Here's how the part is built. I have some questions about the finished solid (model axes, mm). A direction names the side the tool comes from. Coordinates: 2 decimals unless noted, no trailing zeros. Loops run counter-clockwise (first coordinate to the right, second up) from the corner with the lowest first, then second, coordinate; pieces in that order, holes last. Notation, with made-up numbers: (84.5, -1.75) -> (109.5, -1.75) arc R18 ccw to (109.5, 11.25) -> close; hole circle Ø11 at (30, -11). An arc over 180 degrees is marked (long way). Answer as a JSON object with one key per item and string values. Group by question number.
1) I want a section at C-C (z = 4). Count the separate pieces of the cut face and the enclosed holes in it, then the cut area to 3 significant figures.
2) If we mould it in two halves opening along X, with no side actions, what happens to faces 1 (the cylindrical face through (179.66, -8.5, 4.7)), 2 (the flat face through (80, 45, 0)), 3 (the flat face through (75.101, 119, 5))? For each: +X half, -X half, draft (parallel to the pull), parting line (faces both ways), or undercut.
3) I want a section at A-A (x = 172.5). Write out the boundary of the cut face in (y, z) (3 decimals), then the cut area to 3 significant figures.
4) I'm going to push flat-ended pins straight in: pin 1 (4 mm diameter, centred on y = 92.5, z = 5, fed in from -X); pin 2 (7.5 mm diameter, centred on x = -57.29, y = -9.46, fed in from -Z); pin 3 (0.9 mm diameter, centred on y = -45, z = 6.5, fed in from +X); pin 4 (3 mm diameter, centred on x = 120.5, z = 4, fed in from -Y). Where does each tip first touch, or does it pass through?
5) I need wall thicknesses on probe 1 along X at (y, z) = (-7, 6); probe 2 along Y at (x, z) = (83, 1.25); probe 3 along X at (y, z) = (-10, 6). Which ranges of each line are inside material? Lowest first, please. Write a range as [from, to].
6) I want a section at D-D (y = 120). Write out the boundary of the cut face in (x, z) (3 decimals), then the cut area to 3 significant figures.
7) Which directions (+Z, -Z, +X, -X, +Y, -Y) give clear straight access to the entire face, cutting with the end or side of a thin tool? Please do faces 4 (the flat face through (88, -44.322, 5)), 5 (the flat face through (-33, 80.741, 5)), 6 (the flat face through (222.711, 43, 5)).
8) I want a section at B-B (y = 66). Write out the boundary of the cut face in (x, z) (3 decimals).
```python
from build123d import *

# Parameters (mm, degrees)
SKETCH1_R                    = 14.2875
BOSS_EXTRUDE1_DEPTH          = 9.525
SKETCH2_W                    = 285.640227578
SKETCH2_H                    = 77.156349518
CUT_EXTRUDE1_DEPTH           = 267.58430025
SKETCH4_W                    = 213.36
SKETCH4_H                    = 65.465352004
CUT_EXTRUDE2_DEPTH           = 267.58430025
FILLET2_R                    = 25.4
SKETCH16_W                   = 9.525
SKETCH16_H                   = 0.985363282
CUT_EXTRUDE3_DEPTH           = 390.572219806
SKETCH17_W                   = 147.610011278
SKETCH17_H                   = 12.7
CUT_EXTRUDE4_DEPTH           = 267.045158533
TAP_DRILL_FOR_M6X0_75_TAP1_D = 5.25
F_6_4_6_4_DIAMETER_HOLE1_D   = 6.4


with BuildPart() as part:
    # Sketch1 → Boss-Extrude1 (new body)
    with BuildSketch(Plane.XY):
        Polygon((-138.259383474, 48.991487021), (32.210627804, -121.478524257), (222.710627804, -121.478524257), (222.710627804, 146.206839025), (-138.259383474, 146.206839025), align=None)
        with Locations(Location((180.538014078, 76.831975743, 0), (0, 0, 180))):
            Circle(SKETCH1_R, mode=Mode.SUBTRACT)
    extrude(amount=BOSS_EXTRUDE1_DEPTH)

    # Sketch2 → Cut-Extrude1 (cut, through all)
    with BuildSketch(Plane.XY.offset(9.525)):
        with Locations((98.940514015, -82.900349498)):
            Rectangle(SKETCH2_W, SKETCH2_H)
    extrude(amount=-CUT_EXTRUDE1_DEPTH, mode=Mode.SUBTRACT)

    # Sketch4 → Cut-Extrude2 (cut, through all)
    with BuildSketch(Plane.XY.offset(9.525)):
        with Locations((-31.579383474, 113.474163023)):
            Rectangle(SKETCH4_W, SKETCH4_H)
    extrude(amount=-CUT_EXTRUDE2_DEPTH, mode=Mode.SUBTRACT)

    # Fillet2
    fillet2_edges = [part.edges().sort_by_distance(p)[0] for p in [
        (-138.259383474, 80.741487021, 4.7625),
        (75.100616526, 80.741487021, 4.7625),
    ]]
    fillet(fillet2_edges, radius=FILLET2_R)

    # Sketch16 → Cut-Extrude3 (cut, through all)
    with BuildSketch(Plane(origin=(222.710627804, 0, 0), x_dir=(0, 0, -1), z_dir=(1, 0, 0))):
        with Locations((-4.7625, 145.714157384)):
            Rectangle(SKETCH16_W, SKETCH16_H)
    extrude(amount=-CUT_EXTRUDE3_DEPTH, mode=Mode.SUBTRACT)

    # Sketch17 → Cut-Extrude4 (cut, through all)
    with BuildSketch(Plane(origin=(0, 0, 0), x_dir=(-1, 0, 0), z_dir=(0, 0, -1))):
        with Locations((-148.905622165, 138.871475743)):
            Rectangle(SKETCH17_W, SKETCH17_H)
    extrude(amount=-CUT_EXTRUDE4_DEPTH, mode=Mode.SUBTRACT)

    # Tap Drill for M6x0.75 Tap1 (through all)
    with Locations(Plane.XY.offset(9.525)):
        with Locations((208.638014078, 104.931975743), (152.438014078, 104.931975743), (152.438014078, 48.731975743), (208.638014078, 48.731975743)):
            Hole(TAP_DRILL_FOR_M6X0_75_TAP1_D / 2)

    # Ø6.4 (6.4) Diameter Hole1 (through all)
    with Locations(Plane.XY.offset(9.525)):
        with Locations((-57.289372206, -9.464524257), (62.710627794, -9.464524257), (182.710627794, -9.464524257)):
            Hole(F_6_4_6_4_DIAMETER_HOLE1_D / 2)


solid = part.part
```
Determined:
{
 "1": {"separate pieces": "1", "enclosed holes": "8", "area": "47,600 mm^2"},
 "2": {"face 1": "undercut", "face 2": "draft", "face 3": "-X half"},
 "3": {"outline": "(-44.322, 0) -> (65.02, 0) -> (65.02, 9.525) -> (-44.322, 9.525) -> close; (88.644, 0) -> (132.521, 0) -> (132.521, 9.525) -> (88.644, 9.525) -> close", "area": "1,460 mm^2"},
 "4": {"pin 1": "x = 69.71", "pin 2": "z = 0", "pin 3": "x = -43.88", "pin 4": "y = -44.32"},
 "5": {"probe 1": "[-82.27, -59.33], [-55.25, 60.67], [64.75, 180.67], [184.75, 222.71]", "probe 2": "[-44.32, 132.52]", "probe 3": "[-79.27, -60.44], [-54.13, 59.56], [65.87, 179.56], [185.87, 222.71]"},
 "6": {"outline": "(75.101, 0) -> (222.711, 0) -> (222.711, 9.525) -> (75.101, 9.525) -> close", "area": "1,410 mm^2"},
 "7": {"face 4": "+Z, -Z, +X, -Y", "face 5": "+Z, -Z, -X, +Y", "face 6": "+Z, -Z, +X, +Y, -Y"},
 "8": {"outline": "(-135.915, 0) -> (171.221, 0) -> (171.221, 9.525) -> (-135.915, 9.525) -> close; (189.855, 0) -> (222.711, 0) -> (222.711, 9.525) -> (189.855, 9.525) -> close"}
}
